```python
from build123d import *

# Parameters (mm, degrees)
F0_W     = 19.05
F0_H     = 1219.2
F0_W_2   = 323.85
F0_W_3   = 342.9
F1_DEPTH = 19.05
F2_DEPTH = 3.175
F3_W     = 19.05
F3_H     = 1219.2
F4_DEPTH = 3.175


with BuildPart() as f1:
    # F0 (on Front) → F1 (new body)
    with BuildSketch(Plane.XZ):
        with Locations((-451.089586, 158.169563)):
            Rectangle(F0_W, F0_H)
        with Locations((-279.639586, 158.169563)):
            Rectangle(F0_W_2, F0_H)
        with Locations((-108.189586, 158.169563)):
            Rectangle(F0_W, F0_H)
        with Locations((72.785414, 158.169563)):
            Rectangle(F0_W_3, F0_H)
        with Locations((253.760414, 158.169563)):
            Rectangle(F0_W, F0_H)
        with Locations((425.210414, 158.169563)):
            Rectangle(F0_W_2, F0_H)
        with Locations((596.660414, 158.169563)):
            Rectangle(F0_W, F0_H)
    extrude(amount=F1_DEPTH)

    # F0 (on Front) → F2 (cut)
    with BuildSketch(Plane.XZ):
        with Locations((596.660414, 158.169563)):
            Rectangle(F0_W, F0_H)
        with Locations((-451.089586, 158.169563)):
            Rectangle(F0_W, F0_H)
        with Locations((253.760414, 158.169563)):
            Rectangle(F0_W, F0_H)
        with Locations((-108.189586, 158.169563)):
            Rectangle(F0_W, F0_H)
    extrude(amount=F2_DEPTH, mode=Mode.SUBTRACT)

    # F3 (on face) → F4 (cut)
    with BuildSketch(Plane.XZ.offset(19.05)):
        with Locations((596.660414, 158.169563)):
            Rectangle(F3_W, F3_H)
        with Locations((-451.089586, 158.169563)):
            Rectangle(F3_W, F3_H)
        with Locations((-108.189586, 158.169563)):
            Rectangle(F3_W, F3_H)
        with Locations((253.760414, 158.169563)):
            Rectangle(F3_W, F3_H)
    extrude(amount=-F4_DEPTH, mode=Mode.SUBTRACT)


solid = f1.part
```
For this review, take the finished solid that the model builds, in its own axes (mm). Coordinates: 2 decimals unless noted, no trailing zeros. Order: outer loops, then holes, each group sorted by start corner. A loop starts at its lowest first (then second) coordinate and runs counter-clockwise, first axis right, second up. Notation, with made-up numbers: (6, 10) -> (58, 10) arc R20 ccw to (58, 15) -> close; hole circle Ø1 at (0.25, -1.75). An arc over 180 degrees is marked (long way). Answer as CSV lines item,"result".
Q1. Wall thickness on line 1 along X through (y, z) = (-17.25, 676): over which ranges is the line inside the solid? List them lowest first. Write a range as [from, to].
Model answer:
line 1,"x = [-441.56, -117.71], [-98.66, 244.24], [263.29, 587.14]"
Q2. Clearance check with flat-ended pins moving along their axes: pin 1 Ø5.5 at (x, z) = (-110.5, 31) entering from -Y (3 decimals); pin 2 Ø9.5 at (x, z) = (-111, -4) entering from +Y (3 decimals); pin 3 Ø2.5 at (y, z) = (-2, 113) entering from -X; pin 4 Ø2.5 at (y, z) = (-1.5, 417) entering from +X. State where each tip first meets the part, or that it passes through.
Model answer:
pin 1,"stops at y = -15.875"
pin 2,"stops at y = -3.175"
pin 3,"stops at x = -460.61"
pin 4,"stops at x = 587.14"
Q3. We need section A-A (z = 140.5). State the section outline as (x, y) points (3 decimals).
Model answer:
outline,"(-460.615, -15.875) -> (-441.565, -15.875) -> (-441.565, -19.05) -> (-117.715, -19.05) -> (-117.715, -15.875) -> (-98.665, -15.875) -> (-98.665, -19.05) -> (244.235, -19.05) -> (244.235, -15.875) -> (263.285, -15.875) -> (263.285, -19.05) -> (587.135, -19.05) -> (587.135, -15.875) -> (606.185, -15.875) -> (606.185, -3.175) -> (587.135, -3.175) -> (587.135, 0) -> (263.285, 0) -> (263.285, -3.175) -> (244.235, -3.175) -> (244.235, 0) -> (-98.665, 0) -> (-98.665, -3.175) -> (-117.715, -3.175) -> (-117.715, 0) -> (-441.565, 0) -> (-441.565, -3.175) -> (-460.615, -3.175) -> close"
